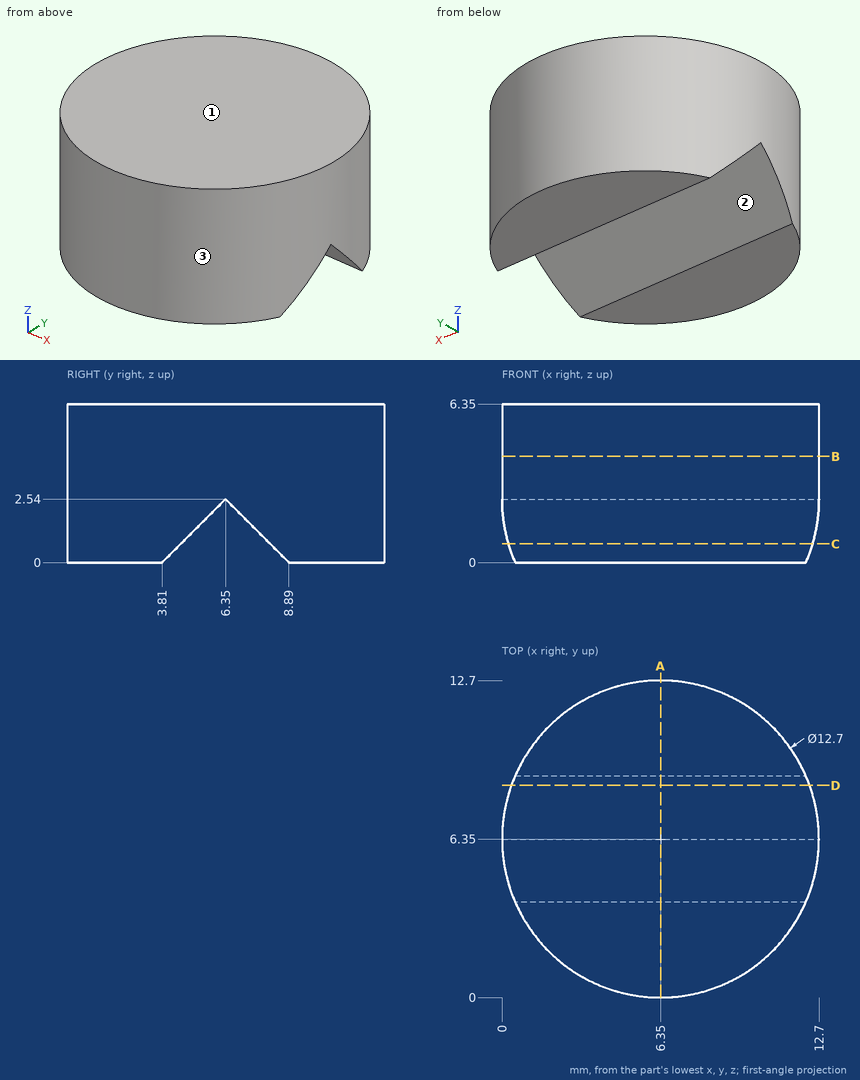
Source: three-view drawing plus pictorial views. Frame: mm from the lowest corner of the part. Coordinates: 2 decimals unless noted, no trailing zeros. Write each loop counter-clockwise with the first axis right and the second up, starting at its lowest first coordinate (ties: lowest second). Pieces come first, ordered by that corner, then holes. Notation, with made-up numbers: (-14, 79.5) -> (23, 79.5) arc R5 ccw to (23, 83.5) -> close; hole circle Ø4 at (26.5, -35). An arc over 180 degrees is marked (long way). Write each question's results on one line, items separated by ' | '.
Item 1: Section query D-D on y = 8.5. Return loops of the section in (x, z).
Conclusion:
outline: (0.38, 0.39) -> (12.32, 0.39) -> (12.32, 6.35) -> (0.38, 6.35) -> close
Item 2: Material intervals for probe 1 along Y at (x, z) = (9, 1); probe 2 along Y at (x, z) = (11.25, 0.5); probe 3 along X at (y, z) = (6.5, 3), sorted ascending.
Conclusion:
probe 1: y = 0.58 to 4.81, 7.89 to 12.12 | probe 2: y = 2.31 to 4.31, 8.39 to 10.39 | probe 3: x = 0 to 12.7
Item 3: Section query C-C on z = 0.75. Return loops of the section in (x, y), plus the area to 3 significant figures.
Conclusion:
outline: (0.26, 4.56) arc R6.35 ccw to (12.44, 4.56) -> close; (0.26, 8.14) -> (12.44, 8.14) arc R6.35 ccw to start | area: 81.8 mm^2
Item 4: Section query A-A on x = 6.35. Return loops of the section in (y, z), plus the area to 3 significant figures.
Conclusion:
outline: (0, 0) -> (3.81, 0) -> (6.35, 2.54) -> (8.89, 0) -> (12.7, 0) -> (12.7, 6.35) -> (0, 6.35) -> close | area: 74.2 mm^2
Item 5: Section query B-B on z = 4.25. Return loops of the section in (x, y), plus the area to 3 significant figures.
Conclusion:
outline: circle Ø12.7 at (6.35, 6.35) | area: 127 mm^2
Item 6: Mould query, pull axis Y, two halves, no side actions, for the marked faces 1, 2 and 3. Classes: +Y half, -Y half, draft (parallel to the pull), parting line (faces both ways), or undercut.
Conclusion:
face 1: draft | face 2: undercut | face 3: parting line
Item 7: Pin query (flat end, axial travel): pin 1 Ø3 at (x, y) = (3.5, 5.5) entering from -Z; pin 2 Ø1 at (x, z) = (5.5, 4.5) entering from +Y; pin 3 Ø1.5 at (x, y) = (10, 6) entering from -Z. Return the tip coordinate at first contact, or that it passes through.
Conclusion:
pin 1: stops at z = 0.19 | pin 2: stops at y = 12.69 | pin 3: stops at z = 1.44
